Autodesk Inventor part; units mm, degrees
ref_plane "YZ Plane" through (0, 0, 0) normal (1, 0, 0) x (0, 1, 0)
ref_plane "XZ Plane" through (0, 0, 0) normal (0, 1, 0) x (-1, 0, 0)
ref_plane "XY Plane" through (0, 0, 0) normal (0, 0, 1) x (1, 0, 0)
sketch "Sketch1" plane through (0, 0, 0) normal (0, 1, 0) x (-1, 0, 0)
  line L0 (0, 0) -> (-100, 0)
  line L1 (-100, 0) -> (-100, -60)
  line L2 (-100, -60) -> (0, -60)
  line L3 (0, -60) -> (0, 0)
  dimension "d2" = 100
  dimension "d3" = 60
extrude "Extrusion1" add sketch "Sketch1" along normal blind 1
sketch "Sketch3" plane through (0, 1, 0) normal (0, 1, 0) x (1, 0, 0)
  circle A0 centre (10.0878, 20.0328) radius 1.5
  circle A1 centre (10.0878, 40.0181) radius 1.5
  point P0 (0, 0)
  dimension "d11" = 3
  dimension "d12" = 3
extrude "Extrusion3" cut sketch "Sketch3" against normal blind 1
sketch "Sketch4" plane through (0, 1, 0) normal (0, 1, 0) x (1, 0, 0)
  point P0 (0, 0)
sketch "Sketch5" plane through (0, 1, 0) normal (0, 1, 0) x (1, 0, 0)
  point P0 (0, 0)
sketch "Sketch6" plane through (0, 1, 0) normal (0, 1, 0) x (1, 0, 0)
  point P0 (0, 0)
sketch "Sketch7" plane through (0, 1, 0) normal (0, 1, 0) x (1, 0, 0)
  circle A0 centre (90.0288, 20.0328) radius 1.5
  circle A1 centre (90.0288, 40.0181) radius 1.5
  point P0 (0, 0)
  dimension "d15" = 3
  dimension "d16" = 3
extrude "Extrusion4" cut sketch "Sketch7" against normal blind 1
properties part number "3dmodelling2"
Input: part model. Units: mm. Frame: model coordinates. Coordinates: 2 decimals unless noted, no trailing zeros.
1. Contact query for a flat-ended pin moving along its axis: P1, Ø2.5, axis at x = 10.09, z = -20.03, coming from the +Y side. Output: stop coordinate, or through.
Checked values:
P1: passes through
2. Draft query along X for faces 1 (the flat face through (51, 0, -30)), 2 (the cylindrical face through (91.414, 0.507, -19.458)), 3 (the cylindrical face through (9.76, 0.51, -18.57)). Return one class per face: +X half, -X half, draft (parallel to the pull), parting line (faces both ways), or undercut.
Checked values:
face 1: draft
face 2: undercut
face 3: undercut
3. Ray query, line 1 along Z through (x, y) = (9, 0.5); line 2 along X through (y, z) = (0.3, -41); line 3 along X through (y, z) = (0.25, -20.5). Return the intervals inside material, ascending.
Checked values:
line 1: z = -60 to -41.05, -38.99 to -21.07, -19 to 0
line 2: x = 0 to 8.95, 11.22 to 88.89, 91.16 to 100
line 3: x = 0 to 8.66, 11.51 to 88.6, 91.45 to 100
